```python
from build123d import *

# Parameters (mm, degrees)
F0_W     = 950
F0_H     = 900
F0_W_2   = 60
F0_H_2   = 60
F1_DEPTH = 40
F2_DEPTH = 400
F3_W     = 60
F3_H     = 1700
F4_DEPTH = 60
F5_DEPTH = 60
F6_W     = 60
F6_H     = 60
F7_DEPTH = 340


# Not quite as in the source:
# - a feature names something its author has since deleted; it is built from what else it names


with BuildPart() as f1:
    # F0 (on Top) → F1 (new body)
    with BuildSketch(Plane.XY):
        with Locations((0, 450)):
            Rectangle(F0_W, F0_H)
        with Locations((-395, 80)):
            Rectangle(F0_W_2, F0_H_2, mode=Mode.SUBTRACT)
        with Locations((395, 80)):
            Rectangle(F0_W_2, F0_H_2, mode=Mode.SUBTRACT)
        with Locations((-395, 820)):
            Rectangle(F0_W_2, F0_H_2, mode=Mode.SUBTRACT)
        with Locations((395, 820)):
            Rectangle(F0_W_2, F0_H_2, mode=Mode.SUBTRACT)
        with Locations((-395, 80)):
            Rectangle(F0_W_2, F0_H_2)
        with Locations((-395, 820)):
            Rectangle(F0_W_2, F0_H_2)
        with Locations((395, 80)):
            Rectangle(F0_W_2, F0_H_2)
        with Locations((395, 820)):
            Rectangle(F0_W_2, F0_H_2)
    extrude(amount=F1_DEPTH)

    # F0 (on Top) → F2 (join)
    with BuildSketch(Plane.XY):
        with Locations((-395, 80)):
            Rectangle(F0_W_2, F0_H_2)
        with Locations((-395, 820)):
            Rectangle(F0_W_2, F0_H_2)
        with Locations((395, 80)):
            Rectangle(F0_W_2, F0_H_2)
        with Locations((395, 820)):
            Rectangle(F0_W_2, F0_H_2)
    extrude(amount=-F2_DEPTH)

    # F3 (on face) → F4 (join)
    with BuildSketch(Plane(origin=(0, 0, 0), x_dir=(1, 0, 0), z_dir=(0, 0, -1))):
        with Locations((-230, -850)):
            Rectangle(F3_W, F3_H)
        with Locations((230, -850)):
            Rectangle(F3_W, F3_H)
    extrude(amount=F4_DEPTH)

    # F3 (on face) → F5 (join)
    with BuildSketch(Plane(origin=(0, 0, 0), x_dir=(1, 0, 0), z_dir=(0, 0, -1))):
        with Locations((-230, -850)):
            Rectangle(F3_W, F3_H)
        with Locations((230, -850)):
            Rectangle(F3_W, F3_H)
    extrude(amount=F5_DEPTH)

    # F6 (on face) → F7 (join)
    with BuildSketch(Plane(origin=(0, 0, -60), x_dir=(1, 0, 0), z_dir=(0, 0, -1))):
        with Locations((230, -1670)):
            Rectangle(F6_W, F6_H)
        with Locations((-230, -1670)):
            Rectangle(F6_W, F6_H)
        with Locations((-230, -30)):
            Rectangle(F6_W, F6_H)
        with Locations((230, -30)):
            Rectangle(F6_W, F6_H)
    extrude(amount=F7_DEPTH)


solid = f1.part
```
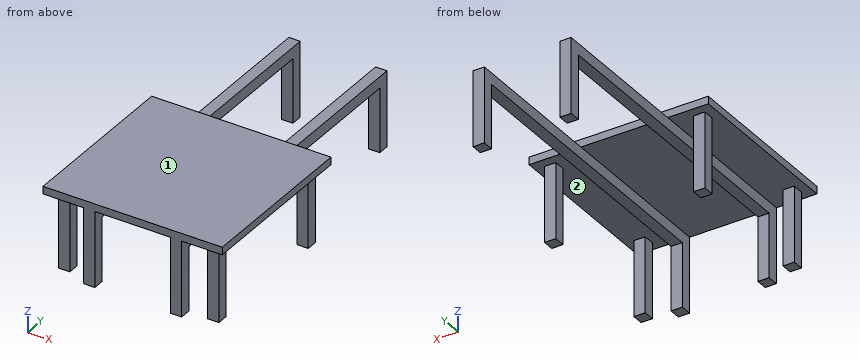
The model under review builds one solid part; all positions refer to its coordinate system, in mm. Face numbers are marked on the shaded views. Round coordinates to 2 decimals unless told otherwise and drop trailing zeros. Write each loop counter-clockwise with the first axis right and the second up, starting at its lowest first coordinate (ties: lowest second). Pieces come first, ordered by that corner, then holes. Notation, with made-up numbers: (50.5, 85.5) -> (79.5, 85.5) arc R21 ccw to (79.5, 120.5) -> close; hole circle Ø2 at (83, 12.25). An arc over 180 degrees is marked (long way). Use CSV: the item, a comma, the result in double quotes.
Q1. Consider section B-B (y = 1235.5). Give the boundary of the cut face in (x, z), then the cut area to 3 significant figures.
Checks:
outline,"(-260, -60) -> (-200, -60) -> (-200, 0) -> (-260, 0) -> close; (200, -60) -> (260, -60) -> (260, 0) -> (200, 0) -> close"
area,"7,200 mm²"
Q2. To check wall thickness, follow probe 1 along X at (y, z) = (1526.5, -34.5); probe 2 along Y at (x, z) = (213.5, -213); probe 3 along X at (y, z) = (849.5, -306.5). State the ranges of each line that lie inside material, in increasing order. Write a range as [from, to].
Checks:
probe 1,"[-260, -200], [200, 260]"
probe 2,"[0, 60], [1640, 1700]"
probe 3,"[-425, -365], [365, 425]"
Q3. Consider section D-D (x = 243). Give the boundary of the cut face in (y, z), then the cut area to 3 significant figures.
Checks:
outline,"(0, -400) -> (60, -400) -> (60, -60) -> (1640, -60) -> (1640, -400) -> (1700, -400) -> (1700, 0) -> (900, 0) -> (900, 40) -> (0, 40) -> close"
area,"179,000 mm²"
Q4. For pin 1 Ø18 at (x, z) = (404.5, -266) entering from +Y; pin 2 Ø20 at (x, z) = (119.5, 23) entering from +Y; pin 3 Ø18 at (x, y) = (-230, 1456.5) entering from +Z, all flat-tipped, find the tip position at first contact; note any pin that passes through.
Checks:
pin 1,"y = 850"
pin 2,"y = 900"
pin 3,"z = 0"
Q5. Consider section C-C (y = 622). Give the boundary of the cut face in (x, z).
Checks:
outline,"(-475, 0) -> (-260, 0) -> (-260, -60) -> (-200, -60) -> (-200, 0) -> (200, 0) -> (200, -60) -> (260, -60) -> (260, 0) -> (475, 0) -> (475, 40) -> (-475, 40) -> close"
Q6. Mouldability with a two-part tool opening along Y and no side actions: class the marked faces 1 and 2 as released by +Y, released by -Y, zero draft, split by the parting line, or undercut.
Checks:
face 1,"zero draft"
face 2,"undercut"
Q7. Consider section A-A (z = -221.5). State how many separate pieces and enclosed holes the cut face has, then the cut area to 3 significant figures.
Checks:
separate pieces,"8"
enclosed holes,"0"
area,"28,800 mm²"
